Answer from the drawing. Dimensions are ordinates in mm from the lowest x, y and z of the part. A direction names the side the tool comes from. Give positions to 0.01 mm unless a question says otherwise; leave off trailing zeros. Loops run counter-clockwise (first coordinate to the right, second up) from the corner with the lowest first, then second, coordinate; pieces in that order, holes last.
(1) Find section A-A, the plane y = 1.75. Write down the section's boundary in (x, z).
(2) Which of the six approach directions +Z, -Z, +X, -X, +Y, -Y give full straight-line access (tool end or side, diameter ignored) to the marked faces 1, 2, 3, 4 and 5?
(3) Each of these flat-tipped pins is pushed along its axis until it touches: P1, Ø1.2, axis at y = 13, z = 4, coming from the -X side (3 decimals); P2, Ø1, axis at x = 5.5, z = 6, coming from the -Y side; P3, Ø1.5, axis at x = 3.5, z = 6, coming from the +Y side. Where does it stop, or does it pass through?
(4) Find section D-D, the plane z = 4. Write down the section's boundary in (x, y) (3 decimals).
(5) Straight lines are drawn through the part: probe 1 along X at (y, z) = (16, 4.25) (3 decimals); probe 2 along X at (y, z) = (13.25, 5.5) (3 decimals); probe 3 along Y at (x, z) = (0.5, 3.75). For each, find the intervals that lie inside material, in ascending order.
(6) Find section B-B, the plane z = 1.46. Write down the section's boundary in (x, y).
(7) Find section C-C, the plane x = 6.54. Write down the section's boundary in (y, z), then the cut area to 3 significant figures.
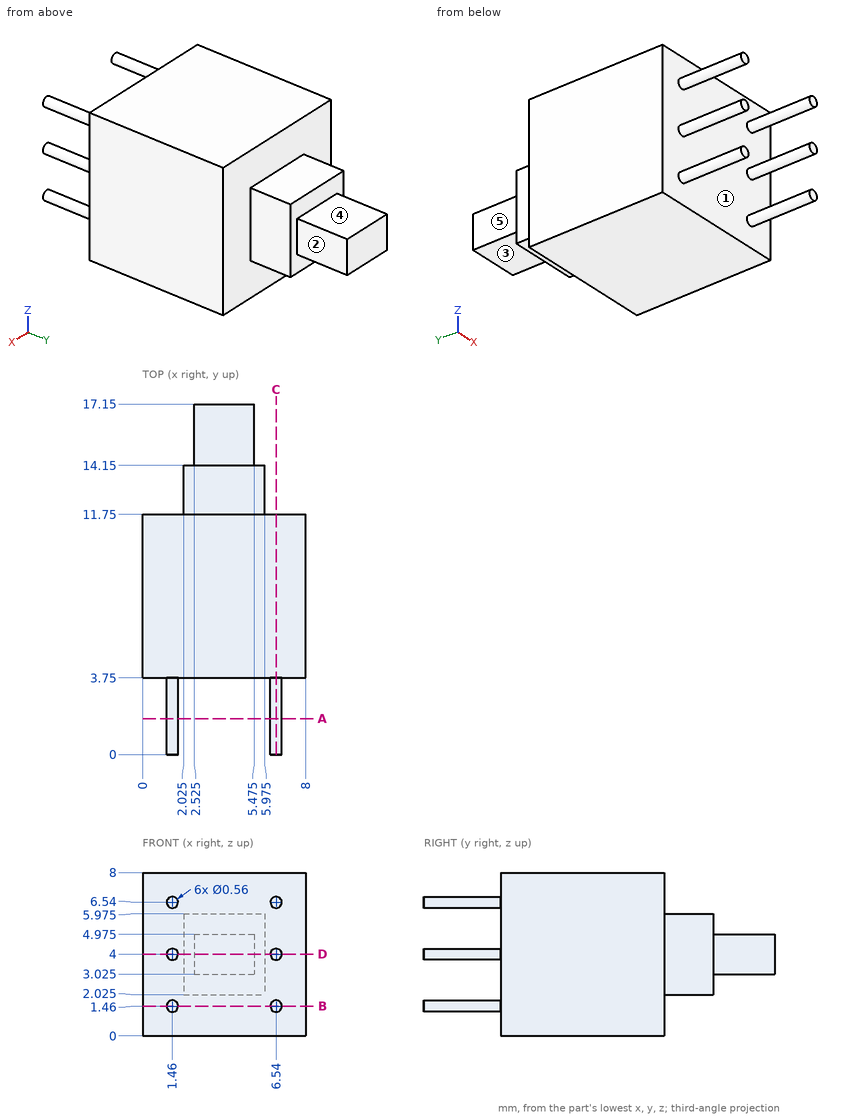
Entries:
1. outline: circle Ø0.56 at (1.46, 1.46); circle Ø0.56 at (1.46, 4); circle Ø0.56 at (1.46, 6.54); circle Ø0.56 at (6.54, 1.46); circle Ø0.56 at (6.54, 4); circle Ø0.56 at (6.54, 6.54)
2. face 1: -Y
2. face 2: +Z, -Z, +X, +Y
2. face 3: -Z, +X, -X, +Y
2. face 4: +Z, +X, -X, +Y
2. face 5: +Z, -Z, -X, +Y
3. P1: stops at x = 2.025
3. P2: stops at y = 3.75
3. P3: stops at y = 14.15
4. outline: (0, 3.75) - (1.18, 3.75) - (1.18, 0) - (1.74, 0) - (1.74, 3.75) - (6.26, 3.75) - (6.26, 0) - (6.82, 0) - (6.82, 3.75) - (8, 3.75) - (8, 11.75) - (5.975, 11.75) - (5.975, 14.15) - (5.475, 14.15) - (5.475, 17.15) - (2.525, 17.15) - (2.525, 14.15) - (2.025, 14.15) - (2.025, 11.75) - (0, 11.75) - close
5. probe 1: x = 2.525 to 5.475
5. probe 2: x = 2.025 to 5.975
5. probe 3: y = 3.75 to 11.75
6. outline: (0, 3.75) - (1.18, 3.75) - (1.18, 0) - (1.74, 0) - (1.74, 3.75) - (6.26, 3.75) - (6.26, 0) - (6.82, 0) - (6.82, 3.75) - (8, 3.75) - (8, 11.75) - (0, 11.75) - close
7. outline: (0, 1.18) - (3.75, 1.18) - (3.75, 0) - (11.75, 0) - (11.75, 8) - (3.75, 8) - (3.75, 6.82) - (0, 6.82) - (0, 6.26) - (3.75, 6.26) - (3.75, 4.28) - (0, 4.28) - (0, 3.72) - (3.75, 3.72) - (3.75, 1.74) - (0, 1.74) - close
7. area: 70.3 mm2
